```python
from build123d import *

# Parameters (mm, degrees)
BOSS_EXTRUDE1_DEPTH = 28
BOSS_EXTRUDE2_START = -10
SKETCH3_W           = 22
SKETCH3_H           = 32
SKETCH3_R           = 3.7
SKETCH3_W_2         = 2
SKETCH3_H_2         = 3
BOSS_EXTRUDE2_DEPTH = 4
CUT_EXTRUDE1_START  = -7
CUT_EXTRUDE1_DEPTH  = 7
CHAMFER1_SIZE       = 10
CHAMFER1_SIZE2      = 5.773502692
CUT_EXTRUDE2_REACH  = 87.346
SKETCH5_W           = 20
SKETCH5_H           = 60
SKETCH6_W           = 23
SKETCH6_H           = 10
SKETCH6_W_2         = 10
SKETCH6_H_2         = 23
BOSS_EXTRUDE3_DEPTH = 28
SKETCH8_R           = 4.1
CUT_EXTRUDE3_DEPTH  = 77.052613367
CHAMFER2_SIZE       = 10


with BuildPart() as part:
    # Sketch2 → Boss-Extrude1 (new body)
    with BuildSketch(Plane(origin=(0, 0, 0), x_dir=(0, 0, -1), z_dir=(1, 0, 0))):
        with BuildLine():
            Line((0, 40), (-30, 40))
            Line((-30, 40), (-30, -30))
            Line((-30, -30), (40, -30))
            Line((40, -30), (40, 0))
            ThreePointArc((40, 0), (28.284271247, 28.284271247), (0, 40))
        make_face()
        with BuildLine():
            Line((-25, 35), (-25, -25))
            Line((-25, -25), (35, -25))
            Line((35, -25), (35, 0))
            ThreePointArc((35, 0), (24.748737342, 24.748737342), (0, 35))
            Line((0, 35), (-25, 35))
        make_face(mode=Mode.SUBTRACT)
    extrude(amount=BOSS_EXTRUDE1_DEPTH)

    # Sketch3 → Boss-Extrude2 (add)
    with BuildSketch(Plane(origin=(28, 0, 0), x_dir=(0, 0, -1), z_dir=(1, 0, 0)).offset(BOSS_EXTRUDE2_START)):
        with Locations((0, -9)):
            Rectangle(SKETCH3_W, SKETCH3_H)
        Circle(SKETCH3_R, mode=Mode.SUBTRACT)
        with Locations((-8.7, 0)):
            Rectangle(SKETCH3_W_2, SKETCH3_H_2, mode=Mode.SUBTRACT)
        with Locations((8.7, 0)):
            Rectangle(SKETCH3_W_2, SKETCH3_H_2, mode=Mode.SUBTRACT)
    extrude(amount=-BOSS_EXTRUDE2_DEPTH)

    # Sketch4 → Cut-Extrude1 (cut)
    with BuildSketch(Plane(origin=(28, 0, 0), x_dir=(0, 0, -1), z_dir=(1, 0, 0)).offset(CUT_EXTRUDE1_START)):
        with BuildLine():
            Line((0, 40), (-7, 40))
            Line((-7, 40), (-7, 35))
            Line((-7, 35), (0, 35))
            ThreePointArc((0, 35), (24.748737342, 24.748737342), (35, 0))
            Line((35, 0), (35, -7))
            Line((35, -7), (40, -7))
            Line((40, -7), (40, 0))
            ThreePointArc((40, 0), (28.284271247, 28.284271247), (0, 40))
        make_face()
    extrude(amount=CUT_EXTRUDE1_DEPTH, mode=Mode.SUBTRACT)

    # Chamfer1
    chamfer1_edges = [part.edges().sort_by_distance(p)[0] for p in [
        (14, -25, 0),
    ]]
    chamfer1_side = [part.faces().sort_by_distance(p)[0] for p in [
        (14, -9.762838276, 0),
    ]]
    chamfer(chamfer1_edges, length=CHAMFER1_SIZE, length2=CHAMFER1_SIZE2, reference=chamfer1_side[0])

    # Sketch5 → Cut-Extrude2 (cut, up to next)
    with BuildSketch(Plane.XY.offset(30), mode=Mode.PRIVATE) as cut_extrude2_sk1:
        with Locations((14, 5)):
            Rectangle(SKETCH5_W, SKETCH5_H)
    cut_extrude2_tool1 = extrude(cut_extrude2_sk1.sketch, amount=-CUT_EXTRUDE2_REACH, mode=Mode.PRIVATE) & part.part
    add(cut_extrude2_tool1.solids().sort_by_distance((14, 5, 30))[0], mode=Mode.SUBTRACT)

    # Sketch6 → Boss-Extrude3 (add)
    with BuildSketch(Plane(origin=(28, 0, 0), x_dir=(0, 0, -1), z_dir=(1, 0, 0))):
        with Locations((-18.5, 45)):
            Rectangle(SKETCH6_W, SKETCH6_H)
        with Locations((45, -18.5)):
            Rectangle(SKETCH6_W_2, SKETCH6_H_2)
    extrude(amount=-BOSS_EXTRUDE3_DEPTH)

    # Sketch8 → Cut-Extrude3 (cut, through all)
    with BuildSketch(Plane(origin=(28, 0, 0), x_dir=(0, 0, -1), z_dir=(1, 0, 0))):
        with Locations((-18.5, 42.5)):
            Circle(SKETCH8_R)
        with Locations((42.5, -18.5)):
            Circle(SKETCH8_R)
    extrude(amount=-CUT_EXTRUDE3_DEPTH, mode=Mode.SUBTRACT)

    # Chamfer2
    chamfer2_edges = [part.edges().sort_by_distance(p)[0] for p in [
        (14, -7, -50),
        (14, 50, 7),
    ]]
    chamfer(chamfer2_edges, length=CHAMFER2_SIZE)


solid = part.part
```
Input: part model. Units: mm. Frame: model coordinates. A direction names the side the tool comes from. Give positions to 0.01 mm unless a question says otherwise; leave off trailing zeros. Order: outer loops, then holes, each group sorted by start corner. A loop starts at its lowest first (then second) coordinate and runs counter-clockwise, first axis right, second up. Notation, with made-up numbers: M 44,-39 L 88,-39 A13 cw 88,-22 Z; hole C 51,52.25 d2. An arc over 180 degrees is marked long. One line per question, with ' | ' between items. Start each with the question number.
1. Pull-direction query (Y, two-part tool) for faces 6 (the face through (10, 40, 3)), 7 (the face through (16, 1.5, 9)), 8 (the face through (21, 25, -25)); classes: released by +Y, released by -Y, zero draft, split by the parting line, or undercut.
2. Section query C-C (y = -11.5). Return the cut outline in (x, z), and give its area (3 significant figures).
3. Section query A-A (x = 22.5). Return the cut outline in (y, z).
4. Material intervals for probe 1 along Y at (x, z) = (20.25, 18.5); probe 2 along Y at (x, z) = (15.6, 0); probe 3 along Z at (x, y) = (15, -17), sorted ascending. Write a range as [from, to].
5. First-contact query: pin 1 Ø5 at (y, z) = (29, -33.5) entering from -X; pin 2 Ø3 at (x, y) = (14.5, -2.5) entering from -Z; pin 3 Ø6 at (x, z) = (21, 10) entering from +Y; pin 4 Ø12 at (y, z) = (0, 0) entering from +X. Flat tips, straight axial feed; report the tip coordinate or a pass-through.
6. Access query for faces 1 (the face through (10, -4, -40)), 2 (the face through (16, 7, 0)), 3 (the face through (11.073, -20.07, 0.154)), 4 (the face through (16, -1.5, -9)), 5 (the face through (20, -25, -2)). Directions: +Z, -Z, +X, -X, +Y, -Y. A direction counts if a zero-diameter tool reaches every point of the face in a straight line with its end or side. Return the directions, or none.
7. Section query D-D (z = -42.5). Return the cut outline in (x, y).
8. Section query B-B (z = 18.5). Return the cut outline in (x, y), and give its area (3 significant figures).
Here are the results:
1) face 6: released by +Y | face 7: undercut | face 8: zero draft
2) outline: M 0,-44.5 L 28,-44.5 L 28,-35 L 0,-35 Z; M 0,25 L 4,25 L 4,30 L 0,30 Z; M 14,-11 L 18,-11 L 18,11 L 14,11 Z; M 24,25 L 28,25 L 28,30 L 24,30 Z | area: 394 mm²
3) outline: M -30,-50 L -17,-50 L -7,-40 L -7,-35 L -25,-35 L -25,30 L -30,30 Z; M 35,7 L 40,7 L 50,17 L 50,30 L 35,30 Z; hole C -18.5,-42.5 d8.2; hole C 42.5,18.5 d8.2
4) probe 1: [-30, -25], [35, 38.4], [46.6, 50] | probe 2: [-30, -3.7], [3.7, 7], [35, 40] | probe 3: [-50, -46.32], [-38.68, -35], [-11, 11]
5) pin 1: through | pin 2: z = -40 | pin 3: y = 46 | pin 4: x = 18
6) face 1: -Z, +X, -X, +Y | face 2: +Z, +X, -X | face 3: +Z, -X | face 4: +X, -X | face 5: none
7) outline: M 0,-30 L 28,-30 L 28,-22.6 L 0,-22.6 Z; M 0,-14.4 L 28,-14.4 L 28,-9.5 L 0,-9.5 Z
8) outline: M 0,-30 L 28,-30 L 28,-25 L 0,-25 Z; M 0,35 L 28,35 L 28,38.4 L 0,38.4 Z; M 0,46.6 L 28,46.6 L 28,50 L 0,50 Z | area: 330 mm²
